Source: CAD feature listing. Evaluate the final solid. Frame: model axes, mm. Face numbers are marked on the shaded views. A direction names the side the tool comes from. Round coordinates to 2 decimals unless told otherwise and drop trailing zeros. Order: outer loops, then holes, each group sorted by start corner. A loop starts at its lowest first (then second) coordinate and runs counter-clockwise, first axis right, second up. Notation, with made-up numbers: (0, 10) -> (27, 10) arc R32 ccw to (27, 47) -> close; hole circle Ø6 at (30, -10.75). An arc over 180 degrees is marked (long way). Write item = value, one per line. Start each with the question number.
(1) Reachability of the marked faces 1 and 2 from +Z, -Z, +X, -X, +Y, -Y: full face, straight path, thin tool, end or side. Return the list, or none.
(2) Cut plane D-D on z = -17. Return the cut outline in (x, y).
(3) Ray query, line 1 (X direction, y = 24, z = 0); line 2 (X direction, y = 12.25, z = 0); line 3 (Y direction, x = -15, z = -2.5). Return the intervals inside material, ascending.
(4) Cut plane A-A on z = 0. Return the cut outline in (x, y).
(5) Cut plane C-C on x = 0. Return the cut outline in (y, z), then the cut area to 3 significant figures.
(6) Contact query for flat-ended pins moving along their axis: pin 1 Ø6 at (y, z) = (12, -6) entering from +X; pin 2 Ø1.5 at (y, z) = (15.5, -4) entering from -X; pin 3 Ø5 at (y, z) = (16, -7) entering from -X. Output: stop coordinate, or through.
(7) Cut plane B-B on y = 22.25. Return the cut outline in (x, z).
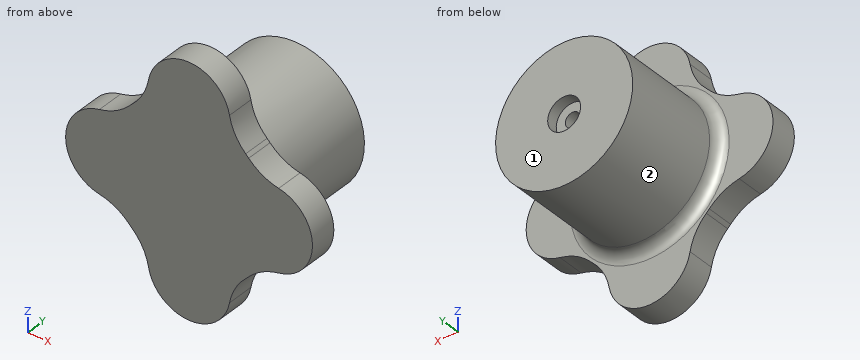
from build123d import *

# Parameters (mm, degrees)
BOSS_EXTRUDE1_DEPTH = 5
FILLET1_R           = 10
SKETCH3_R           = 12.5
BOSS_EXTRUDE2_DEPTH = 20
SKETCH4_R           = 1.35
CUT_EXTRUDE1_DEPTH  = 20
SKETCH5_R           = 3
CUT_EXTRUDE2_DEPTH  = 2
FILLET3_R           = 2


with BuildPart() as part:
    # Sketch2 → Boss-Extrude1 (new body)
    with BuildSketch(Plane(origin=(0, 0, 0), x_dir=(1, 0, 0), z_dir=(0, 1, 0))):
        with BuildLine():
            ThreePointArc((-13.125, -7.261843774), (-10.606601718, -10.606601718), (-7.261843774, -13.125))
            ThreePointArc((-7.261843774, -13.125), (0, -22.5), (7.261843774, -13.125))
            ThreePointArc((7.261843774, -13.125), (10.606601718, -10.606601718), (13.125, -7.261843774))
            ThreePointArc((13.125, -7.261843774), (22.5, 0), (13.125, 7.261843774))
            ThreePointArc((13.125, 7.261843774), (10.606601718, 10.606601718), (7.261843774, 13.125))
            ThreePointArc((7.261843774, 13.125), (0, 22.5), (-7.261843774, 13.125))
            ThreePointArc((-7.261843774, 13.125), (-10.606601718, 10.606601718), (-13.125, 7.261843774))
            ThreePointArc((-13.125, 7.261843774), (-22.5, 0), (-13.125, -7.261843774))
        make_face()
    extrude(amount=BOSS_EXTRUDE1_DEPTH)

    # Fillet1
    fillet1_edges = [part.edges().sort_by_distance(p)[0] for p in [
        (-13.125, 2.5, 7.261843774),
        (-13.125, 2.5, -7.261843774),
        (-7.261843774, 2.5, -13.125),
        (7.261843774, 2.5, -13.125),
        (13.125, 2.5, -7.261843774),
        (13.125, 2.5, 7.261843774),
        (7.261843774, 2.5, 13.125),
        (-7.261843774, 2.5, 13.125),
    ]]
    fillet(fillet1_edges, radius=FILLET1_R)

    # Sketch3 → Boss-Extrude2 (add)
    with BuildSketch(Plane(origin=(0, 5, 0), x_dir=(1, 0, 0), z_dir=(0, 1, 0))):
        with Locations(Location((0, 0, 0), (0, 0, 270))):
            Circle(SKETCH3_R)
    extrude(amount=BOSS_EXTRUDE2_DEPTH)

    # Sketch4 → Cut-Extrude1 (cut)
    with BuildSketch(Plane(origin=(0, 25, 0), x_dir=(1, 0, 0), z_dir=(0, 1, 0))):
        with Locations(Location((0, 0, 0), (0, 0, 270))):
            Circle(SKETCH4_R)
    extrude(amount=-CUT_EXTRUDE1_DEPTH, mode=Mode.SUBTRACT)

    # Sketch5 → Cut-Extrude2 (cut)
    with BuildSketch(Plane(origin=(0, 25, 0), x_dir=(1, 0, 0), z_dir=(0, 1, 0))):
        with Locations(Location((0, 0, 0), (0, 0, 270))):
            Circle(SKETCH5_R)
    extrude(amount=-CUT_EXTRUDE2_DEPTH, mode=Mode.SUBTRACT)

    # Fillet3
    fillet3_edges = [part.edges().sort_by_distance(p)[0] for p in [
        (0, 5, -12.5),
    ]]
    fillet(fillet3_edges, radius=FILLET3_R)


solid = part.part
Evaluation:
q1.face_1 = +Z, -Z, +X, -X, +Y
q1.face_2 = +Y
q2.outline = (-7.23, 0) -> (7.23, 0) -> (7.23, 5) -> (-7.23, 5) -> close
q3.line_1 = -12.5 to -3, 3 to 12.5
q3.line_2 = -12.5 to -1.35, 1.35 to 12.5
q3.line_3 = 0 to 5
q4.outline = (-22.5, 0) -> (22.5, 0) -> (22.5, 5) -> (14.5, 5) arc R2 cw to (12.5, 7) -> (12.5, 25) -> (3, 25) -> (3, 23) -> (1.35, 23) -> (1.35, 5) -> (-1.35, 5) -> (-1.35, 23) -> (-3, 23) -> (-3, 25) -> (-12.5, 25) -> (-12.5, 7) arc R2 cw to (-14.5, 5) -> (-22.5, 5) -> close
q5.outline = (0, -22.5) -> (5, -22.5) -> (5, -14.5) arc R2 cw to (7, -12.5) -> (25, -12.5) -> (25, -3) -> (23, -3) -> (23, -1.35) -> (5, -1.35) -> (5, 1.35) -> (23, 1.35) -> (23, 3) -> (25, 3) -> (25, 12.5) -> (7, 12.5) arc R2 cw to (5, 14.5) -> (5, 22.5) -> (0, 22.5) -> close
q5.area = 666 mm^2
q6.pin_1 = 12.13
q6.pin_2 = -12.07
q6.pin_3 = -11.66
q7.outline = circle Ø25 at (0, 0); hole circle Ø2.7 at (0, 0)
